```python
from build123d import *

# Parameters (mm, degrees)
ESQUISSE1_W        = 250
ESQUISSE1_H        = 116
ESQUISSE1_R        = 40
ESQUISSE1_R_2      = 1.55
ESQUISSE1_W_2      = 15
ESQUISSE1_H_2      = 6
ESQUISSE1_W_3      = 60
ESQUISSE1_H_3      = 3
BOSS_EXTRU_1_DEPTH = 3


with BuildPart() as part:
    # Esquisse1 → Boss.-Extru.1 (new body)
    with BuildSketch(Plane(origin=(0, 0, 0), x_dir=(0, 0, -1), z_dir=(1, 0, 0))):
        with Locations((125, 58)):
            Rectangle(ESQUISSE1_W, ESQUISSE1_H)
        with Locations((125, 58)):
            Circle(ESQUISSE1_R, mode=Mode.SUBTRACT)
        with Locations((125, 103)):
            Circle(ESQUISSE1_R_2, mode=Mode.SUBTRACT)
        with Locations((125, 13)):
            Circle(ESQUISSE1_R_2, mode=Mode.SUBTRACT)
        with Locations((80, 58)):
            Circle(ESQUISSE1_R_2, mode=Mode.SUBTRACT)
        with Locations((170, 58)):
            Circle(ESQUISSE1_R_2, mode=Mode.SUBTRACT)
        with Locations((12.5, 108)):
            Rectangle(ESQUISSE1_W_2, ESQUISSE1_H_2, mode=Mode.SUBTRACT)
        with Locations((12.5, 9)):
            Rectangle(ESQUISSE1_W_2, ESQUISSE1_H_2, mode=Mode.SUBTRACT)
        with Locations((47.5, 108)):
            Rectangle(ESQUISSE1_W_2, ESQUISSE1_H_2, mode=Mode.SUBTRACT)
        with Locations((47.5, 9)):
            Rectangle(ESQUISSE1_W_2, ESQUISSE1_H_2, mode=Mode.SUBTRACT)
        with Locations((100, 112.481116732)):
            Rectangle(ESQUISSE1_W_3, ESQUISSE1_H_3, mode=Mode.SUBTRACT)
        with Locations((200, 112.5)):
            Rectangle(ESQUISSE1_W_3, ESQUISSE1_H_3, mode=Mode.SUBTRACT)
        with Locations((100, 3.518883268)):
            Rectangle(ESQUISSE1_W_3, ESQUISSE1_H_3, mode=Mode.SUBTRACT)
        with Locations((200, 3.5)):
            Rectangle(ESQUISSE1_W_3, ESQUISSE1_H_3, mode=Mode.SUBTRACT)
    extrude(amount=BOSS_EXTRU_1_DEPTH)


solid = part.part
```
Read the model definition and answer for the solid it produces. Units are mm, in the model's axes. Give positions to 0.01 mm unless a question says otherwise; leave off trailing zeros. Order: outer loops, then holes, each group sorted by start corner. A loop starts at its lowest first (then second) coordinate and runs counter-clockwise, first axis right, second up. Notation, with made-up numbers: (61, 53.25) -> (75, 53.25) arc R12 cw to (75, 75.25) -> close; hole circle Ø11 at (59.25, -24.75). An arc over 180 degrees is marked (long way). Write item = value, one per line.
1. A cutting plane is placed at C-C, the plane x = 2.25. Count the separate pieces of the cut face and the enclosed holes in it, and give its area (3 significant figures).
Numbers:
separate_pieces = 1
enclosed_holes = 13
area = 22,900 mm²
2. A cutting plane is placed at B-B, the plane y = 71. Write down the section's boundary in (x, z).
Numbers:
outline = (0, -250) -> (3, -250) -> (3, -162.83) -> (0, -162.83) -> close; (0, -87.17) -> (3, -87.17) -> (3, 0) -> (0, 0) -> close
3. The mould has two halves that part along Y. Classify faces 1 (the face through (1.479, 70.015, -163.153)), 2 (the face through (3, 97, -151)): +Y half, -Y half, draft (parallel to the pull), parting line (faces both ways), or undercut.
Numbers:
face_1 = undercut
face_2 = draft
4. A cutting plane is placed at A-A, the plane z = -223.5. Write down the section's boundary in (x, y).
Numbers:
outline = (0, 0) -> (3, 0) -> (3, 2) -> (0, 2) -> close; (0, 5) -> (3, 5) -> (3, 111) -> (0, 111) -> close; (0, 114) -> (3, 114) -> (3, 116) -> (0, 116) -> close
5. Straight lines are drawn through the part: line 1 along Y through (x, z) = (1.1, -125); line 2 along Y through (x, z) = (1.7, -199); line 3 along Y through (x, z) = (1.85, -80). For each, find the intervals that lie inside material, in ascending order.
Numbers:
line_1 = 0 to 2.02, 5.02 to 11.45, 14.55 to 18, 98 to 101.45, 104.55 to 110.98, 113.98 to 116
line_2 = 0 to 2, 5 to 111, 114 to 116
line_3 = 0 to 2.02, 5.02 to 56.45, 59.55 to 110.98, 113.98 to 116
